Work out the finished part from the listing and answer in its coordinate system (mm). Round coordinates to 2 decimals unless told otherwise and drop trailing zeros. Order: outer loops, then holes, each group sorted by start corner. A loop starts at its lowest first (then second) coordinate and runs counter-clockwise, first axis right, second up. Notation, with made-up numbers: M -24,37 L -9,37 A21 ccw -9,44 Z; hole C 20,46.25 d7. An arc over 180 degrees is marked long. Return JSON: item names as keys, results as strings.
Autodesk Inventor part; units mm, degrees
ref_plane "YZ Plane" through (0, 0, 0) normal (1, 0, 0) x (0, 1, 0)
ref_plane "XZ Plane" through (0, 0, 0) normal (0, 1, 0) x (-1, 0, 0)
ref_plane "XY Plane" through (0, 0, 0) normal (0, 0, 1) x (1, 0, 0)
sketch "Sketch2" plane through (0, 0, 0) normal (0, 1, 0) x (-1, 0, 0)
  line L0 (0, 195.5) -> (-22, 195.5)
  line L1 (-22, -195.5) -> (0, -195.5)
  line L2 (0, -195.5) -> (0, 195.5)
  line L3 (-22, 195.5) -> (-305, 195.5)
  line L4 (-305, 195.5) -> (-305, 173.5)
  line L5 (-305, 173.5) -> (-22, 173.5)
  line L6 (-22, -195.5) -> (-305, -195.5)
  line L7 (-305, -195.5) -> (-305, -173.5)
  line L8 (-305, -173.5) -> (-22, -173.5)
  circle A0 centre (-292.3, 185.5) radius 3.5
  line L9 (-292.3, 185.5) -> (-292.3, 173.5) construction
  line L10 (-289.7, 179.5) -> (-294.9, 179.5)
  line L11 (-294.9, 179.5) -> (-294.9, 173.5)
  line L12 (-294.9, 173.5) -> (-289.7, 173.5)
  line L13 (-289.7, 173.5) -> (-289.7, 179.5)
  circle A1 centre (-199.1, 185.5) radius 3.5
  circle A2 centre (-105.9, 185.5) radius 3.5
  circle A3 centre (-12.7, 185.5) radius 3.5
  line L14 (-22, 195.5) -> (-22, 173.5) construction
  line L15 (0, 0) -> (337.7885, 0) construction
  line L16 (0, 0) -> (-365.548, 0) construction
  line L17 (-22, 173.5) -> (-22, 0)
  line L18 (-22, -173.5) -> (-22, 0)
  circle A4 centre (-292.3, -185.5) radius 3.5
  line L19 (-289.7, -179.5) -> (-294.9, -179.5)
  line L20 (-294.9, -179.5) -> (-294.9, -173.5)
  line L21 (-289.7, -173.5) -> (-289.7, -179.5)
  circle A5 centre (-199.1, -185.5) radius 3.5
  circle A6 centre (-105.9, -185.5) radius 3.5
  circle A7 centre (-12.7, -185.5) radius 3.5
  line L22 (-294.9, -173.5) -> (-289.7, -173.5)
  dimension "d0" = 22
  dimension "d1" = 22
  dimension "d2" = 22
  dimension "d6" = 347
  dimension "d7" = 7
  dimension "d9" = 12.7
  dimension "d10" = 10
  dimension "d11" = 5.2
  dimension "d12" = 6
  dimension "d15" = 93.2
  dimension "d22" = 185.5
  dimension "d23" = 22
  dimension "d24" = 305
  dimension "d29" = 305
extrude "Extrusion2" add sketch "Sketch2" along normal blind 8 contours L2 L1 L6 L7 L8 L20 L19 L21 L18 L17 L5 L13 L10 L11 L4 L3 L0
equation "\"d1\" = d0"
equation "\"d2\" = d0"
equation "\"d15\" = -0.666667 * d9 + 0.333333 * d24"
equation "\"d23\" = d0"
equation "\"d29\" = d24"
properties part number "Top stabiliser"
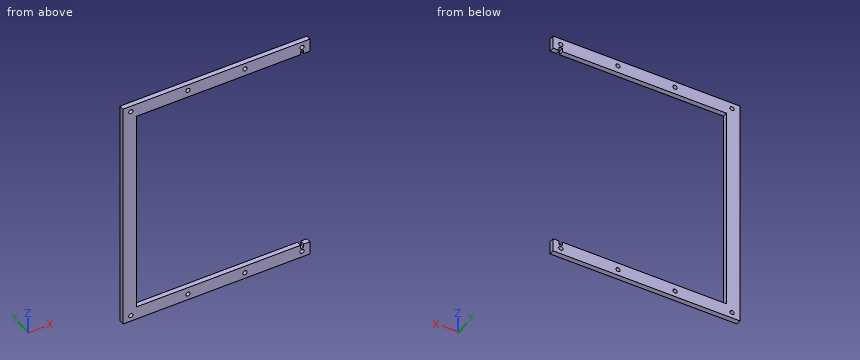
Item 1: Consider line 1 along Z through (x, y) = (199.1, 6.5); line 2 along Z through (x, y) = (292.3, 3); line 3 along X through (y, z) = (6, 185.5). Determine where each line is inside the solid, lowest interval first. Write a range as [from, to].
Output:
{"line 1": "z = [-195.5, -189], [-182, -173.5], [173.5, 182], [189, 195.5]", "line 2": "z = [-195.5, -189], [-182, -179.5], [179.5, 182], [189, 195.5]", "line 3": "x = [0, 9.2], [16.2, 102.4], [109.4, 195.6], [202.6, 288.8], [295.8, 305]"}
Item 2: Find section B-B (x = 239). Determine the outline of the cut face in (y, z), plus the area to 3 significant figures.
Output:
{"outline": "M 0,-195.5 L 8,-195.5 L 8,-173.5 L 0,-173.5 Z; M 0,173.5 L 8,173.5 L 8,195.5 L 0,195.5 Z", "area": "352 mm^2"}
Item 3: Find section C-C (z = -97). Determine the outline of the cut face in (x, y), plus the area to 3 significant figures.
Output:
{"outline": "M 0,0 L 22,0 L 22,8 L 0,8 Z", "area": "176 mm^2"}
Item 4: Find section A-A (y = 2.75). State how many separate pieces and enclosed holes the cut face has, plus the area to 3 significant figures.
Output:
{"separate pieces": "1", "enclosed holes": "8", "area": "20,700 mm^2"}
Item 5: This flat-tipped pin is pushed along its axis until it touches: pin 1 (8 mm diameter, centred on x = 105.9, z = -185.5, fed in from -Y). Where does it stop, or does it pass through?
Output:
{"pin 1": "stops at y = 0"}
